Work out the finished part from the listing and answer in its coordinate system (mm). Face numbers are marked on the shaded views. Round coordinates to 2 decimals unless told otherwise and drop trailing zeros. Order: outer loops, then holes, each group sorted by start corner. A loop starts at its lowest first (then second) coordinate and runs counter-clockwise, first axis right, second up. Notation, with made-up numbers: M 68,1 L 82,1 A17 ccw 82,9 Z; hole C 35.25,8 d10. An arc over 180 degrees is marked long. Return JSON: item names as keys, results as strings.
from build123d import *

# Parameters (mm, degrees)
F1_DEPTH = 4
F2_D     = 3.5


with BuildPart() as f1:
    # F0 (on Front) → F1 (new body)
    with BuildSketch(Plane.XZ):
        with BuildLine():
            ThreePointArc((-5.886911578, 2.4202266574), (-8.8319952599, 0), (-5.886911578, -2.4202266574))
            ThreePointArc((-5.886911578, -2.4202266574), (-6.365, 0), (-5.886911578, 2.4202266574))
        make_face()
        with BuildLine():
            ThreePointArc((-5.886911578, -2.4202266574), (-5.4202243386, -2.1759682794), (-4.9127177697, -2.0349143283))
            ThreePointArc((-4.9127177697, -2.0349143283), (-4.142309561, -1.1443981878), (-3.865, 0))
            ThreePointArc((-3.865, 0), (-4.142309561, 1.1443981878), (-4.9127177697, 2.0349143283))
            ThreePointArc((-4.9127177697, 2.0349143283), (-5.4202243386, 2.1759682794), (-5.886911578, 2.4202266574))
            ThreePointArc((-5.886911578, 2.4202266574), (-6.365, 0), (-5.886911578, -2.4202266574))
        make_face()
        with BuildLine():
            ThreePointArc((4.9127177697, -2.0349143283), (3.865, 0), (4.9127177697, 2.0349143283))
            ThreePointArc((4.9127177697, 2.0349143283), (3.7382668993, 2.1198434614), (2.7329677093, 2.7329677093))
            ThreePointArc((2.7329677093, 2.7329677093), (2.1198434614, 3.7382668993), (2.0349143283, 4.9127177697))
            ThreePointArc((2.0349143283, 4.9127177697), (0, 3.865), (-2.0349143283, 4.9127177697))
            ThreePointArc((-2.0349143283, 4.9127177697), (-2.7329677093, 2.7329677093), (-4.9127177697, 2.0349143283))
            ThreePointArc((-4.9127177697, 2.0349143283), (-4.142309561, 1.1443981878), (-3.865, 0))
            ThreePointArc((-3.865, 0), (-4.142309561, -1.1443981878), (-4.9127177697, -2.0349143283))
            ThreePointArc((-4.9127177697, -2.0349143283), (-2.7329677093, -2.7329677093), (-2.0349143283, -4.9127177697))
            ThreePointArc((-2.0349143283, -4.9127177697), (0, -3.865), (2.0349143283, -4.9127177697))
            ThreePointArc((2.0349143283, -4.9127177697), (2.7329677093, -2.7329677093), (4.9127177697, -2.0349143283))
        make_face()
        with BuildLine():
            ThreePointArc((-2.0349143283, 4.9127177697), (0, 3.865), (2.0349143283, 4.9127177697))
            ThreePointArc((2.0349143283, 4.9127177697), (2.1759682794, 5.4202243386), (2.4202266574, 5.886911578))
            ThreePointArc((2.4202266574, 5.886911578), (0, 6.365), (-2.4202266574, 5.886911578))
            ThreePointArc((-2.4202266574, 5.886911578), (-2.1759682794, 5.4202243386), (-2.0349143283, 4.9127177697))
        make_face()
        with BuildLine():
            ThreePointArc((-2.4202266574, 5.886911578), (0, 6.365), (2.4202266574, 5.886911578))
            ThreePointArc((2.4202266574, 5.886911578), (0, 8.8319952599), (-2.4202266574, 5.886911578))
        make_face()
        with BuildLine():
            ThreePointArc((5.886911578, -2.4202266574), (6.2443341196, -1.23349763), (6.365, 0))
            ThreePointArc((6.365, 0), (6.2443341196, 1.23349763), (5.886911578, 2.4202266574))
            ThreePointArc((5.886911578, 2.4202266574), (5.4202243386, 2.1759682794), (4.9127177697, 2.0349143283))
            ThreePointArc((4.9127177697, 2.0349143283), (3.865, 0), (4.9127177697, -2.0349143283))
            ThreePointArc((4.9127177697, -2.0349143283), (5.4202243386, -2.1759682794), (5.886911578, -2.4202266574))
        make_face()
        with BuildLine():
            ThreePointArc((5.886911578, 2.4202266574), (6.2443341196, 1.23349763), (6.365, 0))
            ThreePointArc((6.365, 0), (6.2443341196, -1.23349763), (5.886911578, -2.4202266574))
            ThreePointArc((5.886911578, -2.4202266574), (8.8319952599, 0), (5.886911578, 2.4202266574))
        make_face()
        with BuildLine():
            ThreePointArc((2.4202266574, -5.886911578), (2.1759682794, -5.4202243386), (2.0349143283, -4.9127177697))
            ThreePointArc((2.0349143283, -4.9127177697), (0, -3.865), (-2.0349143283, -4.9127177697))
            ThreePointArc((-2.0349143283, -4.9127177697), (-2.1759682794, -5.4202243386), (-2.4202266574, -5.886911578))
            ThreePointArc((-2.4202266574, -5.886911578), (0, -6.365), (2.4202266574, -5.886911578))
        make_face()
        with BuildLine():
            ThreePointArc((-2.4202266574, -5.886911578), (0, -8.8319952599), (2.4202266574, -5.886911578))
            ThreePointArc((2.4202266574, -5.886911578), (0, -6.365), (-2.4202266574, -5.886911578))
        make_face()
    extrude(amount=F1_DEPTH)

    # F2 (through all)
    with Locations(Plane(origin=(0, 0, 0), x_dir=(1, 0, 0), z_dir=(0, 1, 0))):
        with Locations((0, 0)):
            Hole(F2_D / 2)


solid = f1.part
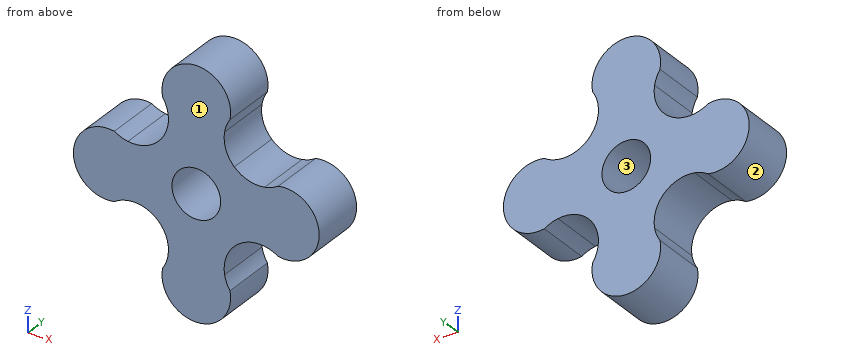
Item 1: Find section A-A (x = 0). Determine the outline of the cut face in (y, z), plus the area to 3 significant figures.
Output:
{"outline": "M -4,-8.83 L 0,-8.83 L 0,-1.75 L -4,-1.75 Z; M -4,1.75 L 0,1.75 L 0,8.83 L -4,8.83 Z", "area": "56.7 mm^2"}
Item 2: Consider line 1 along Z through (x, y) = (4.5, -2.2); line 2 along Z through (x, y) = (-1.5, -3.25); line 3 along Z through (x, y) = (1, -1.5). Determine where each line is inside the solid, lowest interval first. Write a range as [from, to].
Output:
{"line 1": "z = [-2, 2]", "line 2": "z = [-8.32, -0.9], [0.9, 8.32]", "line 3": "z = [-8.62, -1.44], [1.44, 8.62]"}
Item 3: Find section C-C (y = -2.65). Determine the outline of the cut face in (x, z) (3 decimals).
Output:
{"outline": "M -5.887,-2.42 A2.5 cw -2.42,-5.887 A2.467 ccw long 2.42,-5.887 A2.5 cw 5.887,-2.42 A2.467 ccw long 5.887,2.42 A2.5 cw 2.42,5.887 A2.467 ccw long -2.42,5.887 A2.5 cw -5.887,2.42 A2.467 ccw long Z; hole C 0,0 d3.5"}
Item 4: Find section B-B (z = 0). Determine the outline of the cut face in (x, y).
Output:
{"outline": "M -8.83,-4 L -1.75,-4 L -1.75,0 L -8.83,0 Z; M 1.75,-4 L 8.83,-4 L 8.83,0 L 1.75,0 Z"}
Item 5: The mould has two halves that part along Z. Classify the marked faces 1, 2 and 3: pulls with the +Z half, pulls with the -Z half, needs draft (parallel to the pull), parting line crosses it, or undercut.
Output:
{"face 1": "needs draft", "face 2": "parting line crosses it", "face 3": "undercut"}
Item 6: Find section D-D (x = 4.5). Determine the outline of the cut face in (y, z), plus the area to 3 significant figures.
Output:
{"outline": "M -4,-2 L 0,-2 L 0,2 L -4,2 Z", "area": "16.0 mm^2"}
